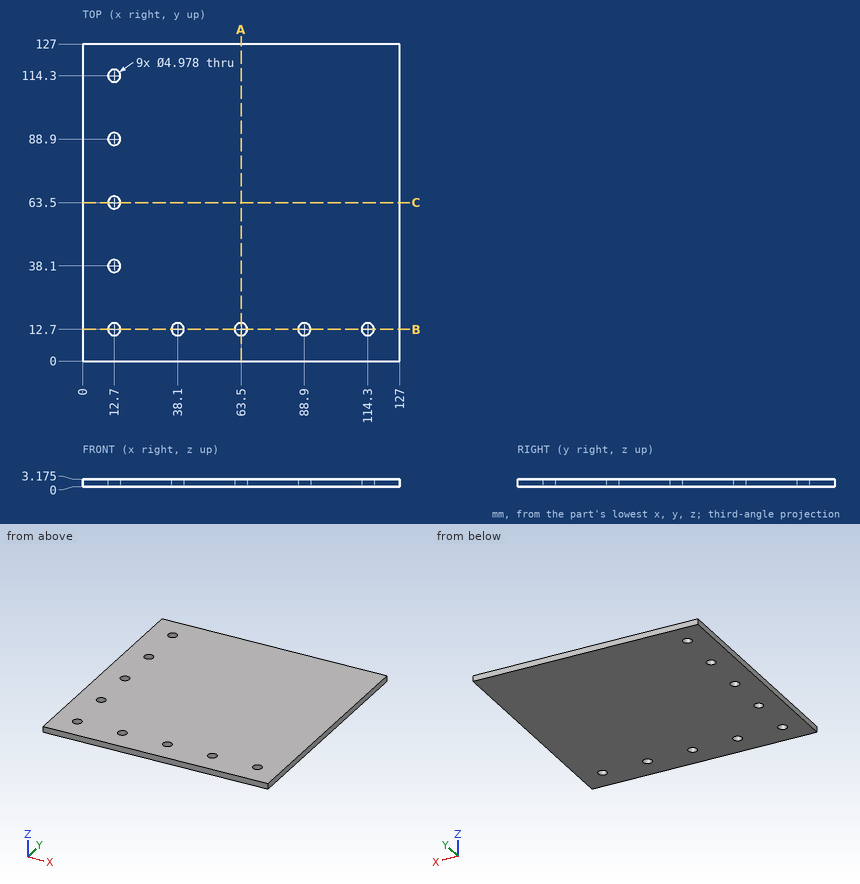
Could you check a few things on this drawing? It's one solid part, dimensions in mm from its lowest x, y, z. Coordinates: 2 decimals unless noted, no trailing zeros. Loops run counter-clockwise (first coordinate to the right, second up) from the corner with the lowest first, then second, coordinate; pieces in that order, holes last.
1. I need wall thicknesses on L1, parallel to Y at x = 12.7, z = 0.9; L2, parallel to X at y = 14, z = 3.05; L3, parallel to Y at x = 38.1, z = 2.4. Which ranges of each line are inside material? Lowest first, please.
2. Imagine slicing it at A-A (x = 63.5). Please give me the cut outline in (y, z) (1 decimal).
3. Imagine slicing it at B-B (y = 12.7). Please give me the cut outline in (x, z) (1 decimal), and give its area (3 significant figures).
Computed values:
1. L1: y = 0 to 10.21, 15.19 to 35.61, 40.59 to 61.01, 65.99 to 86.41, 91.39 to 111.81, 116.79 to 127
1. L2: x = 0 to 10.58, 14.82 to 35.98, 40.22 to 61.38, 65.62 to 86.78, 91.02 to 112.18, 116.42 to 127
1. L3: y = 0 to 10.21, 15.19 to 127
2. outline: (0, 0) - (10.2, 0) - (10.2, 3.2) - (0, 3.2) - close; (15.2, 0) - (127, 0) - (127, 3.2) - (15.2, 3.2) - close
3. outline: (0, 0) - (10.2, 0) - (10.2, 3.2) - (0, 3.2) - close; (15.2, 0) - (35.6, 0) - (35.6, 3.2) - (15.2, 3.2) - close; (40.6, 0) - (61, 0) - (61, 3.2) - (40.6, 3.2) - close; (66, 0) - (86.4, 0) - (86.4, 3.2) - (66, 3.2) - close; (91.4, 0) - (111.8, 0) - (111.8, 3.2) - (91.4, 3.2) - close; (116.8, 0) - (127, 0) - (127, 3.2) - (116.8, 3.2) - close
3. area: 324 mm2
